Design review of the part built by this model. Coordinates are the model's own, in mm. Give positions to 0.01 mm unless a question says otherwise; leave off trailing zeros. Loops run counter-clockwise (first coordinate to the right, second up) from the corner with the lowest first, then second, coordinate; pieces in that order, holes last. Notation, with made-up numbers: (-33.75, 4.25) -> (19.25, 4.25) arc R33 cw to (19.25, 34.25) -> close; hole circle Ø8 at (10.25, 14). An arc over 180 degrees is marked (long way). Answer as CSV lines item,"result".
from build123d import *
from build123d import SkipClean  # not in build123d's __all__

# Parameters (mm, degrees)
F0_W     = 7.9248
F0_H     = 7.9248
F1_DEPTH = 130.175
F2_R     = 1.5875
F3_DEPTH = 25.4
F5_DEPTH = 508


with BuildPart() as f1:
    # F0 (on Front) → F1 (new body)
    with BuildSketch(Plane.XZ):
        Rectangle(F0_W, F0_H)
    extrude(amount=F1_DEPTH)

    # F2 (on face) → F3 (cut)
    with BuildSketch(Plane.YZ.offset(3.9624)):
        with BuildLine():
            ThreePointArc((-125.4125, 0), (-127, 1.5875), (-128.5875, 0))
            ThreePointArc((-128.5875, 0), (-127, -1.5875), (-125.4125, 0))
        make_face()
        with Locations((-3.175, 0)):
            Circle(F2_R)
    extrude(amount=-F3_DEPTH, mode=Mode.SUBTRACT)

    # F4 (on face) → F5 (cut)
    with BuildSketch(Plane(origin=(0, 0, 0), x_dir=(-1, 0, 0), z_dir=(0, 1, 0))):
        with BuildLine():
            ThreePointArc((-3.9624, 0), (-2.8018399098, 2.8018399098), (0, 3.9624))
            Line((0, 3.9624), (-3.9624, 3.9624))
            Line((-3.9624, 3.9624), (-3.9624, 0))
        make_face()
        with BuildLine():
            ThreePointArc((0, 3.9624), (2.8018399098, 2.8018399098), (3.9624, 0))
            Line((3.9624, 0), (3.9624, 3.9624))
            Line((3.9624, 3.9624), (0, 3.9624))
        make_face()
        with BuildLine():
            Line((3.9624, -3.9624), (3.9624, 0))
            ThreePointArc((3.9624, 0), (2.8018399098, -2.8018399098), (0, -3.9624))
            Line((0, -3.9624), (3.9624, -3.9624))
        make_face()
        with BuildLine():
            Line((-3.9624, -3.9624), (0, -3.9624))
            ThreePointArc((0, -3.9624), (-2.8018399098, -2.8018399098), (-3.9624, 0))
            Line((-3.9624, 0), (-3.9624, -3.9624))
        make_face()
    with SkipClean():  # cleaning this boolean's faces spoils the solid; the shape is the same uncleaned
        extrude(amount=-F5_DEPTH, mode=Mode.SUBTRACT)


solid = f1.part
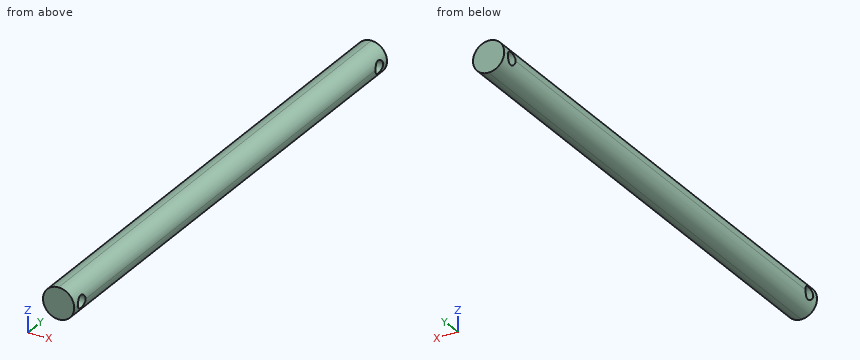
Q1. We need section C-C, the plane y = -58. State the section outline as (x, z) points, and give its area (3 significant figures).
Filled sheet:
outline,"circle Ø7.92 at (0, 0)"
area,"49.3 mm^2"
Q2. We need section A-A, the plane y = -127. State the section outline as (x, z) points.
Filled sheet:
outline,"(-3.63, -1.59) arc R3.96 ccw to (3.63, -1.59) -> close; (-3.63, 1.59) -> (3.63, 1.59) arc R3.96 ccw to start"
Q3. We need section B-B, the plane x = 2.5. State the section outline as (y, z) points (1 decimal), and give its area (3 significant figures).
Filled sheet:
outline,"(-130.2, -3.1) -> (0, -3.1) -> (0, 3.1) -> (-130.2, 3.1) -> close; hole circle Ø3.2 at (-127, 0); hole circle Ø3.2 at (-3.2, 0)"
area,"785 mm^2"
Q4. Clearance check with flat-ended pins moving along their axes: pin 1 Ø3 at (x, y) = (2.5, -39) entering from +Z; pin 2 Ø4 at (y, z) = (-127, 0) entering from -X; pin 3 Ø1.5 at (x, y) = (-2, -95.5) entering from -Z; pin 4 Ø2 at (y, z) = (-47, -2) entering from -X. State where each tip first meets the part, or that it passes through.
Filled sheet:
pin 1,"stops at z = 3.83"
pin 2,"stops at x = -3.96"
pin 3,"stops at z = -3.76"
pin 4,"stops at x = -3.83"
Q5. To check wall thickness, follow probe 1 along Z at (x, y) = (-0.25, -127); probe 2 along Y at (x, z) = (-3.5, -0.5) (3 decimals); probe 3 along Z at (x, y) = (0.25, -71.5). State the ranges of each line that lie inside material, in increasing order. Write a range as from..to.
Filled sheet:
probe 1,"z = -3.95..-1.59, 1.59..3.95"
probe 2,"y = -130.175..-128.507, -125.493..-4.682, -1.668..0"
probe 3,"z = -3.95..3.95"
